The figure shows three views and two pictorial views of one solid part (mm, origin at its lowest corner). Answer the questions. Coordinates: 2 decimals unless noted, no trailing zeros. Order: outer loops, then holes, each group sorted by start corner. A loop starts at its lowest first (then second) coordinate and runs counter-clockwise, first axis right, second up. Notation, with made-up numbers: M 27,74 L 51,74 A13 ccw 51,78 Z; hole C 6,-16 d4. An arc over 180 degrees is marked long. Use a Markdown table: item, result.
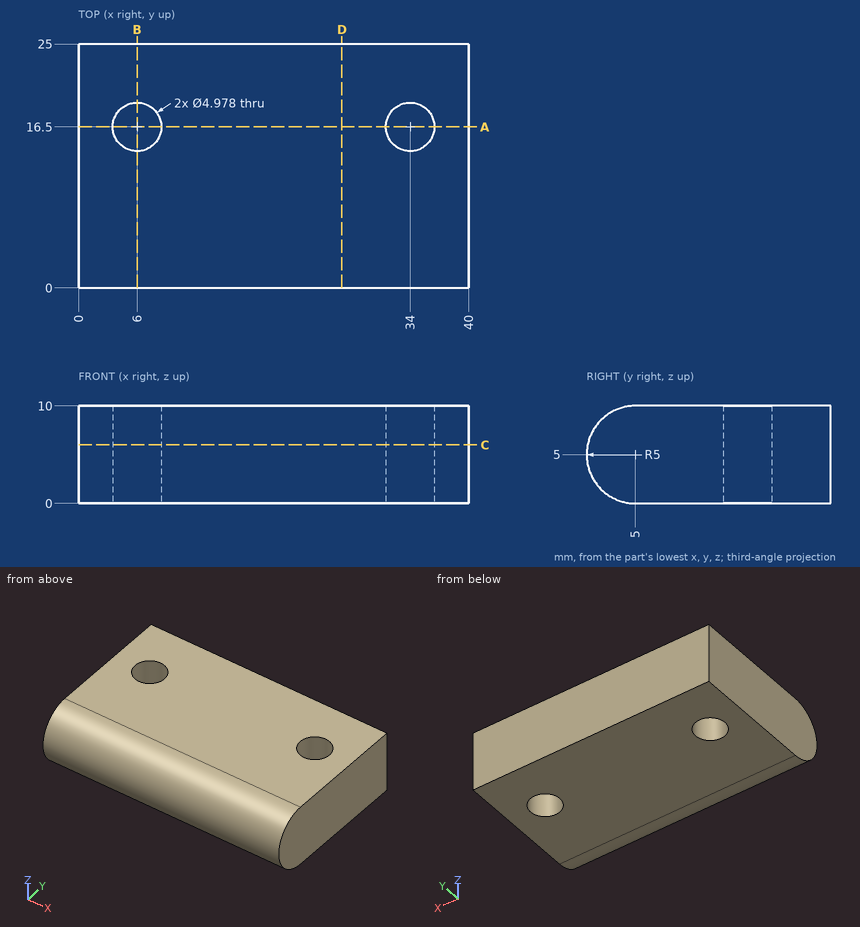
1. Find the intervals of material crossed by probe 1 along X at (y, z) = (17, 4.25); probe 2 along X at (y, z) = (16.75, 4.5); probe 3 along Y at (x, z) = (32.5, 3.75) (1 decimal), in increasing order.
Answers below:
| item | result |
|---|---|
| probe 1 | 0 to 3.56, 8.44 to 31.56, 36.44 to 40 |
| probe 2 | 0 to 3.52, 8.48 to 31.52, 36.48 to 40 |
| probe 3 | 0.2 to 14.5, 18.5 to 25 |
2. Section B-B on x = 6 is taken. Determine the outline of the cut face in (y, z).
Answers below:
| item | result |
|---|---|
| outline | M 5,0 L 14.01,0 L 14.01,10 L 5,10 A5 ccw Z; M 18.99,0 L 25,0 L 25,10 L 18.99,10 Z |
3. A flat-ended cylindrical pin translates along its axis: P1, Ø4, axis at x = 34, y = 16.5, coming from the -Z side. Find the tip coordinate at first contact, or state that the pin passes through.
Answers below:
| item | result |
|---|---|
| P1 | through |
4. Section D-D on x = 27 is taken. Determine the outline of the cut face in (y, z), then the cut area to 3 significant figures.
Answers below:
| item | result |
|---|---|
| outline | M 5,0 L 25,0 L 25,10 L 5,10 A5 ccw Z |
| area | 239 mm² |
5. Section C-C on z = 6 is taken. Determine the outline of the cut face in (x, y), then the cut area to 3 significant figures.
Answers below:
| item | result |
|---|---|
| outline | M 0,0.1 L 40,0.1 L 40,25 L 0,25 Z; hole C 6,16.5 d4.98; hole C 34,16.5 d4.98 |
| area | 957 mm² |
6. Section A-A on y = 16.5 is taken. Determine the outline of the cut face in (x, z).
Answers below:
| item | result |
|---|---|
| outline | M 0,0 L 3.51,0 L 3.51,10 L 0,10 Z; M 8.49,0 L 31.51,0 L 31.51,10 L 8.49,10 Z; M 36.49,0 L 40,0 L 40,10 L 36.49,10 Z |
